Input: part model. Units: mm. Frame: model coordinates. A direction names the side the tool comes from. Round coordinates to 2 decimals unless told otherwise and drop trailing zeros. Loops run counter-clockwise (first coordinate to the right, second up) from the corner with the lowest first, then second, coordinate; pieces in that order, holes last. Notation, with made-up numbers: (-3, -29.75) - (53, -29.75) arc R15 ccw to (53, -20.75) - close; hole circle Ø5 at (65, -14). An arc over 180 degrees is marked (long way). One line per question, with ' | ' between items. Start each with the question number.
Item 1: Material intervals for line 1 along Y through (x, z) = (18.5, 9); line 2 along Z through (x, y) = (6, -2); line 3 along Y through (x, z) = (1.5, 8), sorted ascending.
Item 2: Set-up query: faces 4 (the face through (0, 5.97, 82)), 5 (the face through (-12.624, -17.403, 12.325)), 6 (the face through (12.991, -11.726, 12.325)). Return all of +Z, -Z, +X, -X, +Y, -Y with unobstructed straight access to the full face (end or side cutting, diameter ignored); none if empty.
Item 3: Section C-C, the plane y = 9. Return loops of the section in (x, z).
Item 4: Draft query along Y for faces 1 (the face through (21.384, -2.231, 12.325)), 2 (the face through (10.3, 14.15, 12.32)), 3 (the face through (0, 21.5, 12.3)). Return one class per face: pulls with the +Y half, pulls with the -Y half, needs draft (parallel to the pull), parting line crosses it, or undercut.
Item 5: First-contact query: pin 1 (5 mm diameter, centred on x = -7, z = 24.5, fed in from +Y); pin 2 (3.5 mm diameter, centred on x = -0.5, z = 82, fed in from +Y); pin 3 (6 mm diameter, centred on x = 13.5, y = 11.5, fed in from +Z). Flat tips, straight axial feed; report the tip coordinate or a pass-through.
Item 6: Section D-D, the plane z = 26. Return loops of the section in (x, y).
Item 7: Section A-A, the plane x = 0. Return loops of the section in (y, z).
Item 8: Section B-B, the plane z = 78. Return loops of the section in (x, y), plus the area to 3 significant figures.
```python
from build123d import *

# Parameters (mm, degrees)
SKETCH_2_R               = 17.5
EXTRUDE_2_DEPTH          = 25
EXTRUDE_3_DEPTH          = 25
PATTERN_CIRCULAR_1_COUNT = 15
SKETCH_3_R               = 5
EXTRUDE_4_DEPTH          = 70
EXTRUDE_START            = -26
EXTRUDE_5_DEPTH          = 26


with BuildPart() as part:
    # 草图2 → 凸台-拉伸2 (new body)
    with BuildSketch(Plane.XY):
        Circle(SKETCH_2_R)
    extrude(amount=EXTRUDE_2_DEPTH)

    # 草图4 → 凸台-拉伸3 (add)
    with BuildSketch(Plane(origin=(0, 0, 0), x_dir=(-1, 0, 0), z_dir=(0, 0, -1))):
        with BuildLine():
            ThreePointArc((1.152655242, 21.469079764), (0, 21.5), (-1.152655242, 21.469079764))
            add(Edge.make_bspline(
                [(-2.13271351, 17.369557654), (-2.448019627, 19.937519908), (-1.152655242, 21.469079764)],
                knots=[0, 0, 0, 0.686911927, 0.686911927, 0.686911927], degree=2))
            ThreePointArc((-2.13271351, 17.369557654), (0, 17.5), (2.13271351, 17.369557654))
            add(Edge.make_bspline(
                [(2.13271351, 17.369557654), (2.448019627, 19.937519908), (1.152655242, 21.469079764)],
                knots=[0, 0, 0, 0.686911927, 0.686911927, 0.686911927], degree=2))
        make_face()
    extrude_3 = extrude(amount=-EXTRUDE_3_DEPTH)

    # 阵列(圆周)1: 凸台-拉伸3 ×15 about axis
    pattern_circular_1_axis = Axis((0, 0, 0), (0, 0, 1))
    for i in range(1, PATTERN_CIRCULAR_1_COUNT):
        add(extrude_3.rotate(pattern_circular_1_axis, i * 360 / PATTERN_CIRCULAR_1_COUNT))

    # 草图3 → 凸台-拉伸4 (add)
    with BuildSketch(Plane.XY.offset(25)):
        Circle(SKETCH_3_R)
    extrude(amount=EXTRUDE_4_DEPTH)

    # 草图7 → 凸台-拉伸5 (add)
    with BuildSketch(Plane.XY.offset(95).offset(EXTRUDE_START)):
        with BuildLine():
            Line((1.5, 4.769696007), (1.5, 5.969696007))
            Line((1.5, 5.969696007), (-1.5, 5.969696007))
            Line((-1.5, 5.969696007), (-1.5, 4.769696007))
            ThreePointArc((-1.5, 4.769696007), (0, 5), (1.5, 4.769696007))
        make_face()
    extrude(amount=EXTRUDE_5_DEPTH)


solid = part.part
```
Return value:
1) line 1: -10.95 to -8.54, -4.13 to 0.26, 3.72 to 8.04 | line 2: 0 to 25 | line 3: -17.44 to 20.99
2) face 4: +Z, +X, -X, +Y | face 5: +Z, -Z, -X, -Y | face 6: +Z, -Z
3) outline: (-15.01, 0) - (15.01, 0) - (15.01, 25) - (-15.01, 25) - close
4) face 1: pulls with the -Y half | face 2: undercut | face 3: pulls with the +Y half
5) pin 1: y = 20.08 | pin 2: y = 5.97 | pin 3: z = 25
6) outline: circle Ø10 at (0, 0)
7) outline: (-17.5, 0) - (21.5, 0) - (21.5, 25) - (5, 25) - (5, 69) - (5.97, 69) - (5.97, 95) - (-5, 95) - (-5, 25) - (-17.5, 25) - close
8) outline: (-1.5, 4.77) arc R5 ccw (long way) to (1.5, 4.77) - (1.5, 5.97) - (-1.5, 5.97) - close | area: 81.7 mm2
